Geometry check sheet. Reference: the model listing, model coordinates, mm. Round coordinates to 2 decimals unless told otherwise and drop trailing zeros. Write each loop counter-clockwise with the first axis right and the second up, starting at its lowest first coordinate (ties: lowest second). Pieces come first, ordered by that corner, then holes.
Item 1: Depth check by flat-ended pin: P1, Ø4, axis at y = -1, z = -9.5, coming from the -X side; P2, Ø1, axis at y = -3, z = -5, coming from the +X side; P3, Ø4, axis at x = 10, y = -2, coming from the -Z side; P4, Ø4, axis at x = -12, z = 24.5, coming from the +Y side. Enter the tip coordinate at first touch or a pass-through.
Item 2: Cross-section at C-C (x = -17). State how many separate pieces and enclosed holes the cut face has, then the cut area to 3 significant figures.
Item 3: Scan lines: probe 1 along Z at (x, y) = (0, -2.25); probe 2 along Z at (x, y) = (-4.5, -5.5); probe 3 along X at (y, z) = (-1.5, -20.5). Record each from-to range of solid material in increasing order.
Item 4: Cross-section at D-D (x = 38). Enter the section's corners in (y, z), then the cut area to 3 significant figures.
Item 5: Draft check along Z on faces 1 (the face through (35, -6.77, -21)), 2 (the face through (36.48, -5.13, -12.69)), 3 (the face through (14.446, -3.122, 7.917)). Enter one of: pulls with the +Z half, pulls with the -Z half, needs draft (parallel to the pull), parting line crosses it, or undercut.
Item 6: Cross-section at B-B (x = -36.5). Enter the section's corners in (y, z), then the cut area to 3 significant figures.
Item 7: Cross-section at A-A (y = -4.5). Enter the section's corners in (x, z).
from build123d import *

# Parameters (mm, degrees)
F0_R         = 10.49
F1_DEPTH     = 6.77
F2_T1_DEPTH  = 53.6924086999
F2_T3_DEPTH  = 53.6924086999
F2_T5_DEPTH  = 53.6924086999
F2_T7_DEPTH  = 53.6924086999
F2_T9_DEPTH  = 53.6924086999
F2_T11_DEPTH = 53.6924086999
F2_T14_ANGLE = 273.6993702429
F2_T16_ANGLE = 273.6993702429
F2_T18_ANGLE = 273.6993702439
F2_T20_ANGLE = 273.6993702429
F2_T22_ANGLE = 273.6993702429
F2_T24_ANGLE = 273.6993702429


# Not quite as in the source:
# - a fillet or chamfer that OpenCascade refuses, or shapes differently, is made with other operations: its cross-section is extruded or revolved along the edge and cut away or added


with BuildPart() as f1:
    # F0 (on Front) → F1 (new body)
    with BuildSketch(Plane.XZ):
        with BuildLine():
            Line((18.4621305086, 22.5221560266), (0.4319489998, 54.3327168478))
            Line((0.4319489998, 54.3327168478), (-18.1017140256, 22.8128412157))
            ThreePointArc((-18.1017140256, 22.8128412157), (-14.313385988, 18.9790663983), (-12.9287692735, 13.7702186154))
            ThreePointArc((-12.9287692735, 13.7702186154), (-18.2099214906, 4.66483533), (-28.7358245213, 4.7275960151))
            Line((-28.7358245213, 4.7275960151), (-47.2694875467, -26.792279617))
            Line((-47.2694875467, -26.792279617), (-10.7056430125, -27.0829648061))
            ThreePointArc((-10.7056430125, -27.0829648061), (-0.1742773616, -16.6764412961), (10.2740255001, -27.1663584239))
            ThreePointArc((10.2740255001, -27.1663584239), (10.2739426279, -27.2080555622), (10.2736940127, -27.2497520417))
            Line((10.2736940127, -27.2497520417), (46.8375385469, -27.5404372308))
            Line((46.8375385469, -27.5404372308), (28.8073570381, 4.2701235904))
            ThreePointArc((28.8073570381, 4.2701235904), (14.5087275553, 8.2235265437), (18.4621305086, 22.5221560266))
        make_face()
        with Locations((-23.6347437733, -13.3961398085)):
            Circle(F0_R, mode=Mode.SUBTRACT)
        Circle(F0_R, mode=Mode.SUBTRACT)
        with Locations((23.4187692735, -13.7702186154)):
            Circle(F0_R, mode=Mode.SUBTRACT)
        with Locations((0.2159744999, 27.1663584239)):
            Circle(F0_R, mode=Mode.SUBTRACT)
    extrude(amount=F1_DEPTH)

    # F2: chamfer of 3.33 on 18 edges, made by hand

    # F2_s2 → F2_t1 (cut)
    with BuildSketch(Plane(origin=(-0.9763794466, 0, -1.6605113995), x_dir=(0, 1, 0), z_dir=(-0.5068689464, 0, -0.8620231268))):
        Polygon((-6.77, -23.8372169167), (-3.44, -27.1672169167), (-6.77, -27.1672169167), align=None)
        Polygon((-3.33, -27.1672169167), (0, -23.8372169167), (0, -27.1672169167), align=None)
    extrude(amount=F2_T1_DEPTH, mode=Mode.SUBTRACT)

    # F2_s4 → F2_t3 (cut)
    with BuildSketch(Plane(origin=(28.1913940744, 0, 47.9446094332), x_dir=(0, 1, 0), z_dir=(-0.5068689464, 0, -0.8620231268))):
        Polygon((-6.77, -23.8372169167), (-3.44, -27.1672169167), (-6.77, -27.1672169167), align=None)
        Polygon((-3.33, -27.1672169167), (0, -23.8372169167), (0, -27.1672169167), align=None)
    extrude(amount=F2_T3_DEPTH, mode=Mode.SUBTRACT)

    # F2_s6 → F2_t5 (cut)
    with BuildSketch(Plane(origin=(-0.9498553319, 0, 1.6758251042), x_dir=(0, 1, 0), z_dir=(-0.4930994533, 0, 0.8699729474))):
        Polygon((-6.77, -23.8372169167), (-3.44, -27.1672169167), (-6.77, -27.1672169167), align=None)
        Polygon((-3.33, -27.1672169167), (0, -23.8372169167), (0, -27.1672169167), align=None)
    extrude(amount=F2_T5_DEPTH, mode=Mode.SUBTRACT)

    # F2_s8 → F2_t7 (cut)
    with BuildSketch(Plane(origin=(-55.6169467809, 0, 0.4421587199), x_dir=(0, 1, 0), z_dir=(0.9999683997, 0, -0.0079498206))):
        Polygon((-6.77, -23.8372169167), (-3.44, -27.1672169167), (-6.77, -27.1672169167), align=None)
        Polygon((-3.33, -27.1672169167), (0, -23.8372169167), (0, -27.1672169167), align=None)
    extrude(amount=F2_T7_DEPTH, mode=Mode.SUBTRACT)

    # F2_s10 → F2_t9 (cut)
    with BuildSketch(Plane(origin=(1.9262347785, 0, -0.0153137048), x_dir=(0, 1, 0), z_dir=(0.9999683997, 0, -0.0079498206))):
        Polygon((-3.44, -27.1672169167), (-6.77, -23.8372169167), (-6.77, -27.1672169167), align=None)
        Polygon((-3.33, -27.1672169167), (0, -23.8372169167), (0, -27.1672169167), align=None)
    extrude(amount=F2_T9_DEPTH, mode=Mode.SUBTRACT)

    # F2_s12 → F2_t11 (cut)
    with BuildSketch(Plane(origin=(27.4255527065, 0, -48.3867681532), x_dir=(0, 1, 0), z_dir=(-0.4930994533, 0, 0.8699729474))):
        Polygon((-6.77, -23.8372169167), (-3.44, -27.1672169167), (-6.77, -27.1672169167), align=None)
        Polygon((0, -23.8372169167), (-3.33, -27.1672169167), (0, -27.1672169167), align=None)
    extrude(amount=F2_T11_DEPTH, mode=Mode.SUBTRACT)

    # F2_s13 → F2_t14 (revolve, cut)
    with BuildSketch(Plane(origin=(-4.0831164566, 0, 18.1258589444), x_dir=(0, 1, 0), z_dir=(-0.2197579888, 0, 0.97555442))):
        Polygon((-6.77, 33.6401683275), (-3.44, 30.3101683275), (-6.77, 30.3101683275), align=None)
    revolve(axis=Axis((-23.4187692735, -6.77, 13.7702186154), (0, -1, 0)), revolution_arc=F2_T14_ANGLE, mode=Mode.SUBTRACT)

    # F2_s15 → F2_t16 (revolve, cut)
    with BuildSketch(Plane(origin=(4.3707858991, 0, 18.0586498137), x_dir=(0, 1, 0), z_dir=(0.2352406866, 0, 0.9719371479))):
        Polygon((-6.77, -33.6401683275), (-3.44, -30.3101683275), (-6.77, -30.3101683275), align=None)
    revolve(axis=Axis((23.6347437733, -6.77, 13.3961398085), (0, 1, 0)), revolution_arc=F2_T16_ANGLE, mode=Mode.SUBTRACT)

    # F2_s17 → F2_t18 (revolve, cut)
    with BuildSketch(Plane(origin=(-13.6558960829, 0, -12.59901205), x_dir=(0, 1, 0), z_dir=(-0.7349759161, 0, -0.678093211))):
        Polygon((-6.77, 33.6401683276), (-3.44, 30.3101683277), (-6.77, 30.3101683276), align=None)
    revolve(axis=Axis((-0.2159744998, -6.77, -27.1663584239), (0, -1, 0)), revolution_arc=F2_T18_ANGLE, mode=Mode.SUBTRACT)

    # F2_s19 → F2_t20 (revolve, cut)
    with BuildSketch(Plane(origin=(-17.8246424463, 0, -5.2441132837), x_dir=(0, 1, 0), z_dir=(-0.9593426042, 0, -0.2822441634))):
        Polygon((-3.33, -30.3101683275), (0, -33.6401683275), (0, -30.3101683275), align=None)
    revolve(axis=Axis((-23.4187692735, 0, 13.7702186154), (0, 1, 0)), revolution_arc=F2_T20_ANGLE, mode=Mode.SUBTRACT)

    # F2_s21 → F2_t22 (revolve, cut)
    with BuildSketch(Plane(origin=(13.4538565472, 0, -12.81453653), x_dir=(0, 1, 0), z_dir=(0.7241019176, 0, -0.6896929845))):
        Polygon((0, -33.6401683275), (-3.33, -30.3101683275), (0, -30.3101683275), align=None)
    revolve(axis=Axis((-0.2159744999, 0, -27.1663584239), (0, 1, 0)), revolution_arc=F2_T22_ANGLE, mode=Mode.SUBTRACT)

    # F2_s23 → F2_t24 (revolve, cut)
    with BuildSketch(Plane(origin=(4.3707858991, 0, 18.0586498137), x_dir=(0, 1, 0), z_dir=(0.2352406866, 0, 0.9719371479))):
        Polygon((-3.33, -30.3101683275), (0, -33.6401683275), (0, -30.3101683275), align=None)
    revolve(axis=Axis((23.6347437733, 0, 13.3961398085), (0, 1, 0)), revolution_arc=F2_T24_ANGLE, mode=Mode.SUBTRACT)


solid = f1.part
Resolved:
1. P1: stops at x = -37
1. P2: stops at x = 34.27
1. P3: stops at z = -27.26
1. P4: stops at y = 0
2. separate pieces: 3
2. enclosed holes: 0
2. area: 88.0 mm2
3. probe 1: z = -15.6 to -10.49, 10.49 to 16.68, 37.65 to 51.47
3. probe 2: z = -15.37 to -9.48, 9.48 to 17.8, 36.54 to 41.88
3. probe 3: x = -41.45 to -31.35, -15.92 to -10.58, 10.14 to 15.37, 31.47 to 40.74
4. outline: (-6.77, -24.14) - (-3.44, -27.47) - (-3.33, -27.47) - (0, -24.14) - (0, -18.7) - (-3.33, -11.95) - (-3.44, -11.95) - (-6.77, -18.7) - close
4. area: 71.5 mm2
5. face 1: needs draft
5. face 2: pulls with the +Z half
5. face 3: undercut
6. outline: (-6.77, -23.55) - (-3.44, -26.88) - (-3.33, -26.88) - (0, -23.55) - (0, -15.05) - (-3.33, -8.48) - (-3.44, -8.48) - (-6.77, -15.05) - close
6. area: 91.6 mm2
7. outline: (-45.43, -25.75) - (-11.71, -26.01) arc R11.55 cw to (11.29, -26.2) - (45.01, -26.47) - (28.38, 2.87) arc R11.55 cw to (17.04, 22.88) - (0.42, 52.21) - (-16.68, 23.15) arc R11.55 cw to (-28.33, 3.32) - close; hole circle Ø20.98 at (-23.63, -13.4); hole circle Ø20.98 at (0, 0); hole circle Ø20.98 at (0.22, 27.17); hole circle Ø20.98 at (23.42, -13.77)
